Part model, mm, in its own coordinate system. A direction names the side the tool comes from. Round coordinates to 2 decimals unless told otherwise and drop trailing zeros. Loops run counter-clockwise (first coordinate to the right, second up) from the corner with the lowest first, then second, coordinate; pieces in that order, holes last. Notation, with made-up numbers: M 74,62 L 109,62 A13 ccw 109,77 Z; hole C 0,46 d9. An arc over 180 degrees is marked long. Put each result on its own line as item: value. Start each with the question number.
1) Slice it at C-C on y = 336.55. Give the cut face in (x, z), then the cut area to 3 significant figures.
2) Slice it at A-A on z = -103. Give the cut face in (x, y), then the cut area to 3 significant figures.
3) Probe line 1 along Z through (x, y) = (187, 237); line 2 along X through (y, z) = (304.5, -444); line 3 along Y through (x, z) = (27, -367). List the from-to ranges inside material, lowest first.
4) Drop a flat-ended pin along its axis: pin 1 Ø5 at (y, z) = (223, -194.5) entering from -X. Give the stop position or say it passes through.
5) Slice it at D-D on y = 174.5. Give the cut face in (x, z).
6) Slice it at B-B on x = 183. Give the cut face in (y, z), then the cut area to 3 significant figures.
7) Pull direction Z, two halves, no side cores. Call faces 3 (the flat face through (180, 180, -622.3)), 4 (the flat face through (172, 175, -615.95)), 5 (the flat face through (175, 175, 0)), 6 (the flat face through (349.25, 175, -307)): +Z half, -Z half, draft (parallel to the pull), parting line (faces both ways), or undercut.
8) Which spindle directions (+Z, -Z, +X, -X, +Y, -Y) get a long thin tool onto all of the face, cutting with end or side? Do faces 1 (the cylindrical face through (18.573, 347.259, -315.417)), 2 (the flat face through (355.6, 175, -307)). Say none if no direction does.
```python
from build123d import *

# Parameters (mm, degrees)
SKETCH1_W           = 355.6
SKETCH1_H           = 622.3
BOSS_EXTRUDE1_DEPTH = 355.6
SHELL1_T            = -6.35
SKETCH2_R           = 12.7
BOSS_EXTRUDE2_DEPTH = 622.3


with BuildPart() as part:
    # Sketch1 → Boss-Extrude1 (new body)
    with BuildSketch(Plane(origin=(0, 0, 0), x_dir=(1, 0, 0), z_dir=(0, 1, 0))):
        with Locations((177.8, 311.15)):
            Rectangle(SKETCH1_W, SKETCH1_H)
    extrude(amount=BOSS_EXTRUDE1_DEPTH)

    # Shell1
    shell1_openings = [part.faces().sort_by_distance(p)[0] for p in [
        (177.8, 355.6, -311.15),
        (177.8, 0, -311.15),
        (0, 177.8, -311.15),
    ]]
    offset(amount=SHELL1_T, openings=shell1_openings, kind=Kind.INTERSECTION)

    # Sketch2 → Boss-Extrude2 (add)
    with BuildSketch(Plane(origin=(0, 0, -622.3), x_dir=(-1, 0, 0), z_dir=(0, 0, -1))):
        with Locations((-152.4, 336.55)):
            Circle(SKETCH2_R)
        with Locations((-25.4, 336.55)):
            Circle(SKETCH2_R)
    extrude(amount=-BOSS_EXTRUDE2_DEPTH)


solid = part.part
```
Recorded:
1. outline: M 0,-622.3 L 355.6,-622.3 L 355.6,0 L 0,0 L 0,-6.35 L 12.7,-6.35 L 12.7,-615.95 L 0,-615.95 Z; hole M 38.1,-615.95 L 139.7,-615.95 L 139.7,-6.35 L 38.1,-6.35 Z; hole M 165.1,-615.95 L 349.25,-615.95 L 349.25,-6.35 L 165.1,-6.35 Z
1. area: 39,400 mm2
2. outline: C 25.4,336.55 d25.4; C 152.4,336.55 d25.4; M 349.25,0 L 355.6,0 L 355.6,355.6 L 349.25,355.6 Z
2. area: 3,270 mm2
3. line 1: z = -622.3 to -615.95, -6.35 to 0
3. line 2: x = 349.25 to 355.6
3. line 3: y = 323.95 to 349.15
4. pin 1: stops at x = 349.25
5. outline: M 0,-622.3 L 355.6,-622.3 L 355.6,0 L 0,0 L 0,-6.35 L 349.25,-6.35 L 349.25,-615.95 L 0,-615.95 Z
6. outline: M 0,-622.3 L 355.6,-622.3 L 355.6,-615.95 L 0,-615.95 Z; M 0,-6.35 L 355.6,-6.35 L 355.6,0 L 0,0 Z
6. area: 4,520 mm2
7. face 3: -Z half
7. face 4: undercut
7. face 5: +Z half
7. face 6: undercut
8. face 1: none
8. face 2: +Z, -Z, +X, +Y, -Y
